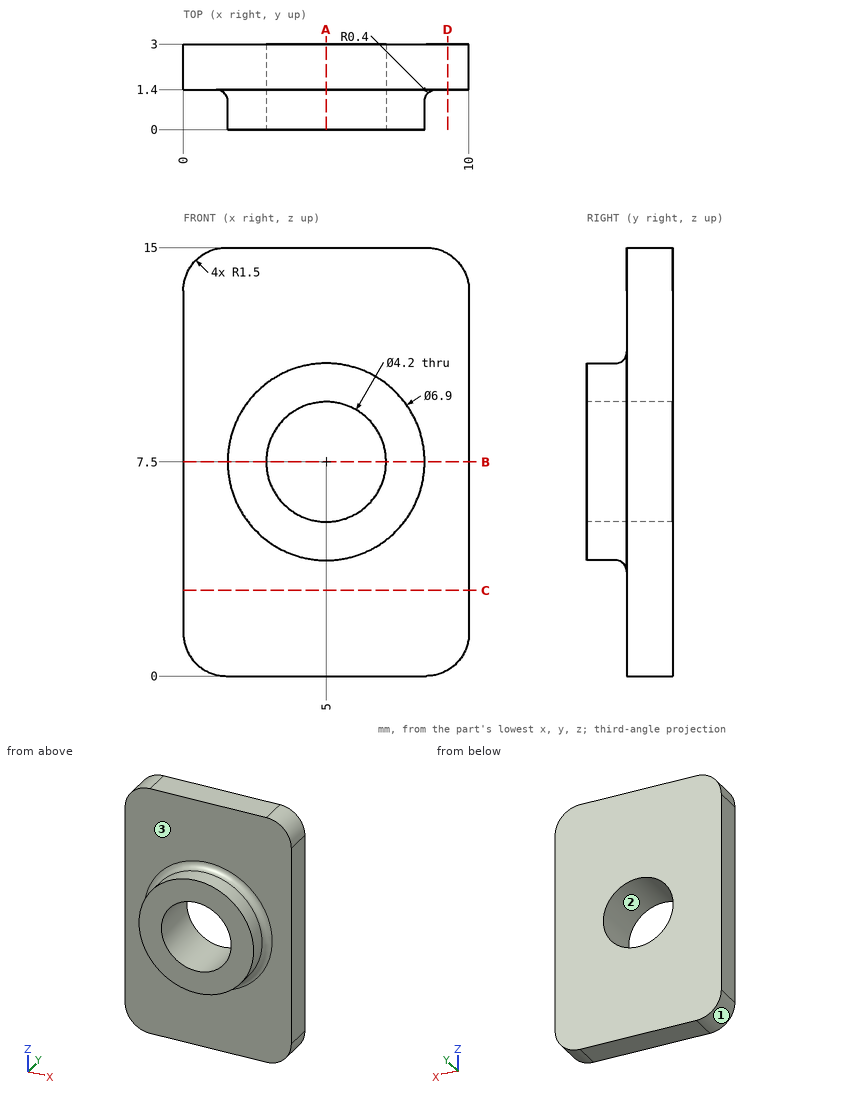
Drawing for the job (mm, zero at the part's lowest x, y, z). Give positions to 0.01 mm unless a question says otherwise; leave off trailing zeros. Loops run counter-clockwise (first coordinate to the right, second up) from the corner with the lowest first, then second, coordinate; pieces in that order, holes last.
1) Band-saw the part on D-D on x = 9.25. List the corners of the cut face in (y, z), then the cut area to 3 significant figures.
Values follow:
outline: (1.4, 0.2) - (3, 0.2) - (3, 14.8) - (1.4, 14.8) - close
area: 23.4 mm2
2) Band-saw the part on B-B on z = 7.5. List the corners of the cut face in (x, y).
Values follow:
outline: (0, 1.4) - (1.15, 1.4) arc R0.4 cw to (1.55, 1) - (1.55, 0) - (2.9, 0) - (2.9, 3) - (0, 3) - close; (7.1, 0) - (8.45, 0) - (8.45, 1) arc R0.4 cw to (8.85, 1.4) - (10, 1.4) - (10, 3) - (7.1, 3) - close
3) Probe line 1 along Z through (x, y) = (5, 1.65); line 2 along Y through (x, z) = (9.75, 8); line 3 along X through (y, z) = (0.45, 8.5). List the from-to ranges inside material, lowest first.
Values follow:
line 1: z = 0 to 5.4, 9.6 to 15
line 2: y = 1.4 to 3
line 3: x = 1.7 to 3.15, 6.85 to 8.3
4) Two-plate mould, pull along X, no slides. Class the marked faces 1, 2 and 3: released by +X, released by -X, zero draft, split by the parting line, or undercut.
Values follow:
face 1: released by -X
face 2: undercut
face 3: zero draft
5) Band-saw the part on A-A on x = 5. List the corners of the cut face in (y, z).
Values follow:
outline: (0, 4.05) - (1, 4.05) arc R0.4 cw to (1.4, 3.65) - (1.4, 0) - (3, 0) - (3, 5.4) - (0, 5.4) - close; (0, 9.6) - (3, 9.6) - (3, 15) - (1.4, 15) - (1.4, 11.35) arc R0.4 cw to (1, 10.95) - (0, 10.95) - close
6) Band-saw the part on C-C on z = 3. List the corners of the cut face in (x, y).
Values follow:
outline: (0, 1.4) - (10, 1.4) - (10, 3) - (0, 3) - close
